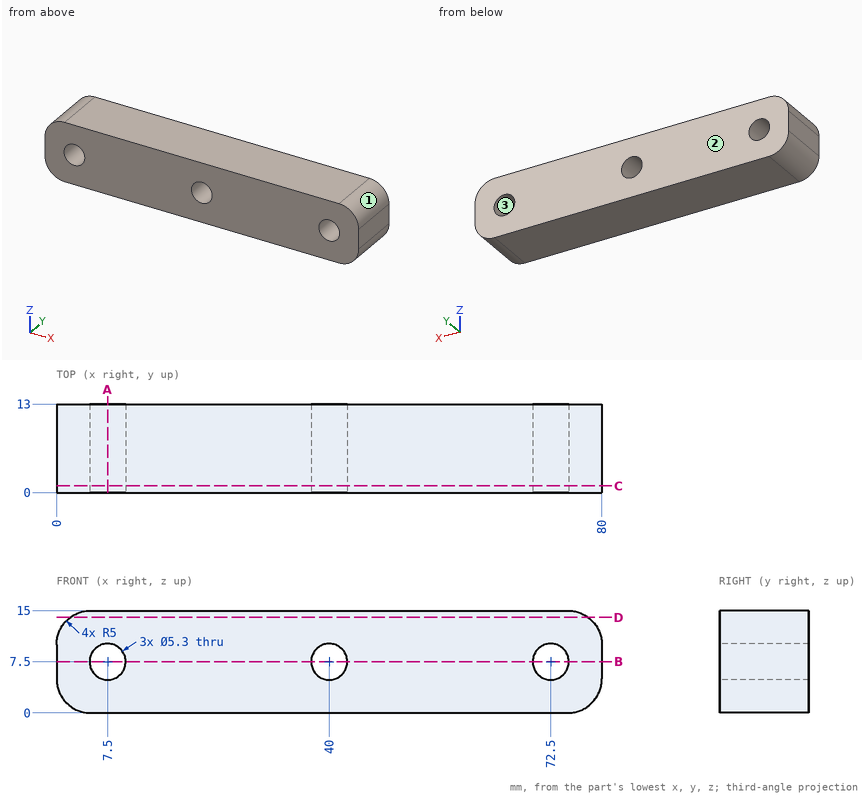
Drawing for the job (mm, zero at the part's lowest x, y, z). Round coordinates to 2 decimals unless told otherwise and drop trailing zeros. Order: outer loops, then holes, each group sorted by start corner. A loop starts at its lowest first (then second) coordinate and runs counter-clockwise, first axis right, second up. Notation, with made-up numbers: (-35.75, 12) -> (1.25, 12) arc R18 ccw to (1.25, 22) -> close; hole circle Ø2 at (14, 69.25). An arc over 180 degrees is marked (long way). Write item = value, one per line. Start each with the question number.
(1) Cut at A-A, the plane x = 7.5. List the corners of the cut face in (y, z).
(2) Pull direction X, two halves, no side cores. Call the marked faces 1, 2 and 3: released by +X, released by -X, zero draft, split by the parting line, or undercut.
(3) Cut at D-D, the plane z = 14. List the corners of the cut face in (x, y), then the cut area to 3 significant figures.
(4) Pin check, flat tip, straight feed: P1, Ø2, axis at y = 9.5, z = 13, coming from the -X side. Stop position of the tip, or through.
(5) Probe line 1 (X direction, y = 6.75, z = 7.5); line 2 (Z direction, x = 72, y = 1); line 3 (X direction, y = 6.5, z = 11.5). List the from-to ranges inside material, lowest first. Write a range as [from, to].
(6) Cut at C-C, the plane y = 1. List the corners of the cut face in (x, z), then the cut area to 3 significant figures.
(7) Cut at B-B, the plane z = 7.5. List the corners of the cut face in (x, y).
Model answer:
q1.outline = (0, 0) -> (13, 0) -> (13, 4.85) -> (0, 4.85) -> close; (0, 10.15) -> (13, 10.15) -> (13, 15) -> (0, 15) -> close
q2.face_1 = released by +X
q2.face_2 = zero draft
q2.face_3 = undercut
q3.outline = (2, 0) -> (78, 0) -> (78, 13) -> (2, 13) -> close
q3.area = 988 mm2
q4.P1 = 0.42
q5.line_1 = [0, 4.85], [10.15, 37.35], [42.65, 69.85], [75.15, 80]
q5.line_2 = [0, 4.9], [10.1, 15]
q5.line_3 = [0.23, 79.77]
q6.outline = (0, 5) arc R5 ccw to (5, 0) -> (75, 0) arc R5 ccw to (80, 5) -> (80, 10) arc R5 ccw to (75, 15) -> (5, 15) arc R5 ccw to (0, 10) -> close; hole circle Ø5.3 at (7.5, 7.5); hole circle Ø5.3 at (40, 7.5); hole circle Ø5.3 at (72.5, 7.5)
q6.area = 1,110 mm2
q7.outline = (0, 0) -> (4.85, 0) -> (4.85, 13) -> (0, 13) -> close; (10.15, 0) -> (37.35, 0) -> (37.35, 13) -> (10.15, 13) -> close; (42.65, 0) -> (69.85, 0) -> (69.85, 13) -> (42.65, 13) -> close; (75.15, 0) -> (80, 0) -> (80, 13) -> (75.15, 13) -> close
